Here's the drawing with two shaded views (mm, measured from the low corner). I have some questions. A direction names the side the tool comes from. Give positions to 0.01 mm unless a question says otherwise; leave off trailing zeros. Order: outer loops, then holes, each group sorted by start corner. A loop starts at its lowest first (then second) coordinate and runs counter-clockwise, first axis right, second up. Notation, with made-up numbers: M 86,-38.75 L 96,-38.75 A18 cw 96,-4.75 Z; hole C -30,-5.75 d4. An arc over 180 degrees is marked long. One line per question, with ' | ' between items. Start each with the question number.
1) For the marked faces 1 and 2, which set-ups out of +Z, -Z, +X, -X, +Y, -Y let a thin tool reach every point of the face, with its end or its side?
2) If we section it at B-B, the plane y = 27.5: Please give me the cut outline in (x, z).
3) Please list where these lines run through material, in increasing order: line 1 along Z through (x, y) = (9.5, 30.5); line 2 along Z through (x, y) = (53, 57); line 3 along Y through (x, z) = (26.5, 23). Write a range as [from, to].
4) If we section it at A-A, the plane z = 45: Please give me the cut outline in (x, y).
5) I'm going to push flat-ended pins straight in: pin 1 Ø6 at (y, z) = (21, 49.5) entering from -X; pin 2 Ø6 at (x, y) = (62, 26.5) entering from +Z; pin 3 Ø6 at (y, z) = (20.5, 25.5) entering from +X. Where does each tip first touch, or does it pass through?
6) Thinking about a two-plate mould opening in X: for the marked faces 3, 4 and 5, which applies, +X half, -X half, draft (parallel to the pull), parting line (faces both ways), or undercut?
7) If we section it at C-C, the plane x = 42.5: Please give me the cut outline in (y, z) (3 decimals).
8) If we section it at D-D, the plane x = 62: Please give me the cut outline in (y, z), plus the area to 3 significant figures.
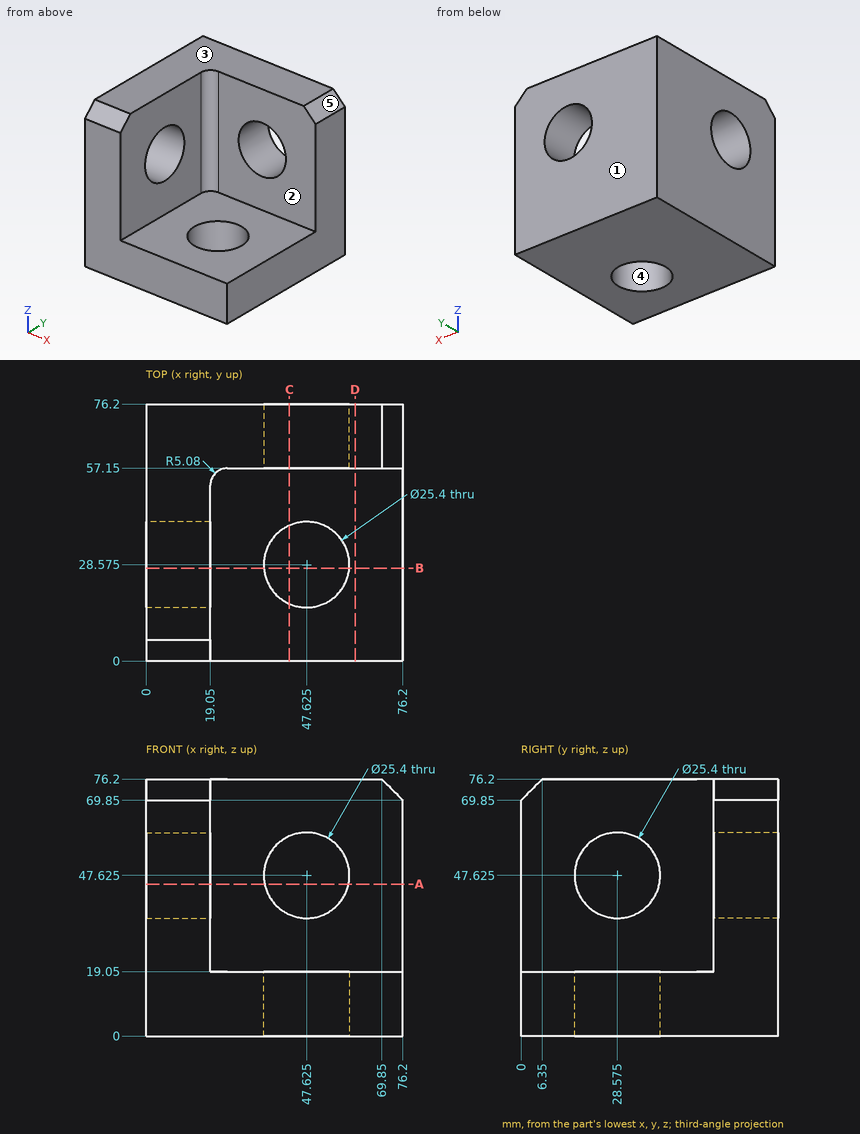
Results found:
1) face 1: +Z, -Z, +X, -X, +Y | face 2: +Z, +X, -Y
2) outline: M 0,0 L 34.97,0 L 34.97,19.05 L 19.05,19.05 L 19.05,34.97 L 0,34.97 Z; M 0,60.28 L 19.05,60.28 L 19.05,76.2 L 0,76.2 Z; M 60.28,0 L 76.2,0 L 76.2,19.05 L 60.28,19.05 Z
3) line 1: z = [0, 35.07], [60.18, 76.2] | line 2: z = [0, 19.05] | line 3: y = [57.15, 76.2]
4) outline: M 0,0 L 19.05,0 L 19.05,16.15 L 0,16.15 Z; M 0,41 L 19.05,41 L 19.05,52.07 A5.08 cw 24.13,57.15 L 35.2,57.15 L 35.2,76.2 L 0,76.2 Z; M 60.05,57.15 L 76.2,57.15 L 76.2,76.2 L 60.05,76.2 Z
5) pin 1: passes through | pin 2: stops at z = 19.05 | pin 3: stops at x = 19.05
6) face 3: draft | face 4: undercut | face 5: +X half
7) outline: M 0,0 L 16.955,0 L 16.955,19.05 L 0,19.05 Z; M 40.195,0 L 76.2,0 L 76.2,36.005 L 57.15,36.005 L 57.15,19.05 L 40.195,19.05 Z; M 57.15,59.245 L 76.2,59.245 L 76.2,76.2 L 57.15,76.2 Z
8) outline: M 0,0 L 76.2,0 L 76.2,76.2 L 57.15,76.2 L 57.15,19.05 L 0,19.05 Z | area: 2,540 mm²
